Design review of the part shown in the three views and the two pictorial views. Dimensions are in mm from the part's minimum x, y and z. Coordinates: 2 decimals unless noted, no trailing zeros. Loops run counter-clockwise (first coordinate to the right, second up) from the corner with the lowest first, then second, coordinate; pieces in that order, holes last.
Q1. For P1, Ø1.5, axis at x = 8.5, y = 2.5, coming from the -Z side; P2, Ø2.5, axis at x = 29, z = 15, coming from the +Y side, all flat-tipped, find the tip position at first contact; note any pin that passes through.
Q2. Add section B-B on y = 1.3. Give the boundary of the cut face in (x, z).
Q3. Add section C-C on x = 3. Give the boundary of the cut face in (y, z).
Q4. Add section A-A on z = 15. Give the boundary of the cut face in (x, y), and give its area (3 significant figures).
Q5. Add section D-D on z = 9.75. Give the boundary of the cut face in (x, y), and give its area (3 significant figures).
Q6. Wall thickness on probe 1 along Z at (x, y) = (29, 2.65); probe 2 along Z at (x, y) = (2, 2.8); probe 3 along Y at (x, z) = (16, 1): over which ranges is each line inside the solid? List them lowest first.
Q7. Draft analysis for pull direction Z (two halves, no side actions). For the marked faces 1, 2 and 3, state which applies: released by +Z, released by -Z, zero draft, split by the parting line, or undercut.
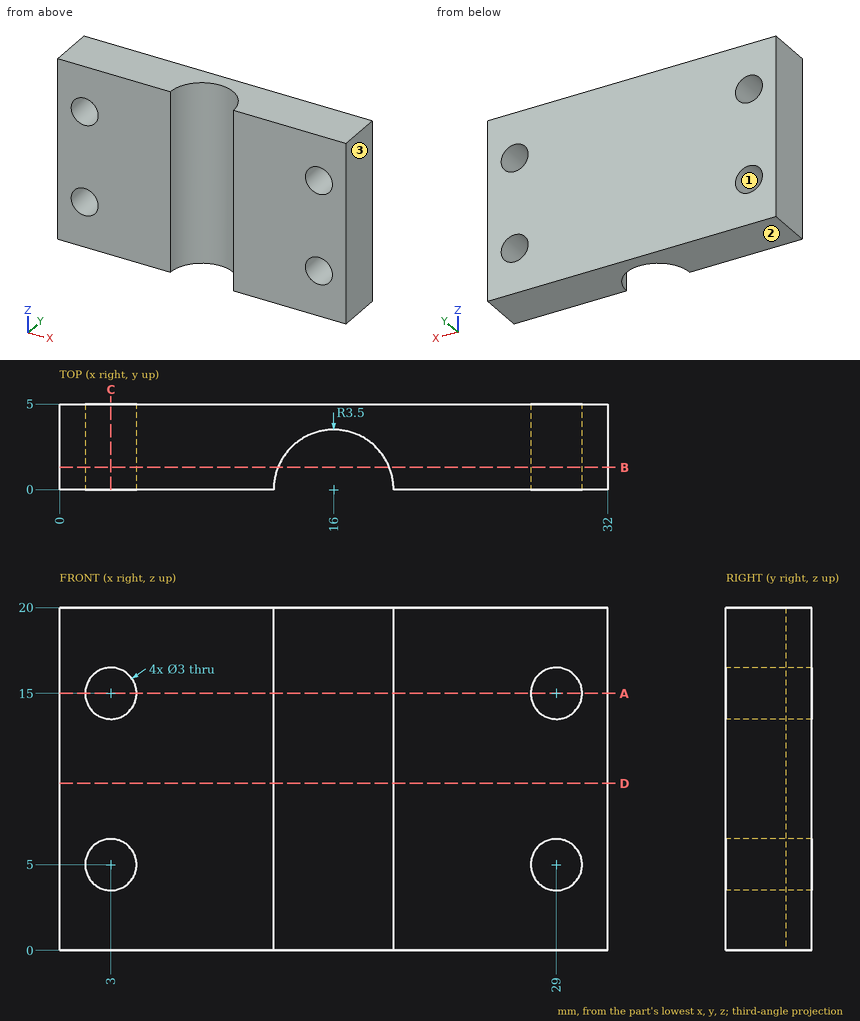
Entries:
1. P1: stops at z = 0
1. P2: passes through
2. outline: (0, 0) - (12.75, 0) - (12.75, 20) - (0, 20) - close; (19.25, 0) - (32, 0) - (32, 20) - (19.25, 20) - close; hole circle Ø3 at (3, 5); hole circle Ø3 at (3, 15); hole circle Ø3 at (29, 5); hole circle Ø3 at (29, 15)
3. outline: (0, 0) - (5, 0) - (5, 3.5) - (0, 3.5) - close; (0, 6.5) - (5, 6.5) - (5, 13.5) - (0, 13.5) - close; (0, 16.5) - (5, 16.5) - (5, 20) - (0, 20) - close
4. outline: (0, 0) - (1.5, 0) - (1.5, 5) - (0, 5) - close; (4.5, 0) - (12.5, 0) arc R3.5 cw to (19.5, 0) - (27.5, 0) - (27.5, 5) - (4.5, 5) - close; (30.5, 0) - (32, 0) - (32, 5) - (30.5, 5) - close
4. area: 111 mm2
5. outline: (0, 0) - (12.5, 0) arc R3.5 cw to (19.5, 0) - (32, 0) - (32, 5) - (0, 5) - close
5. area: 141 mm2
6. probe 1: z = 0 to 3.5, 6.5 to 13.5, 16.5 to 20
6. probe 2: z = 0 to 3.88, 6.12 to 13.88, 16.12 to 20
6. probe 3: y = 3.5 to 5
7. face 1: undercut
7. face 2: released by -Z
7. face 3: zero draft
